Answer from the drawing. Dimensions are ordinates in mm from the lowest x, y and z of the part. Give positions to 0.01 mm unless a question says otherwise; leave off trailing zeros. Order: outer loops, then holes, each group sorted by start corner. A loop starts at its lowest first (then second) coordinate and runs counter-clockwise, first axis right, second up.
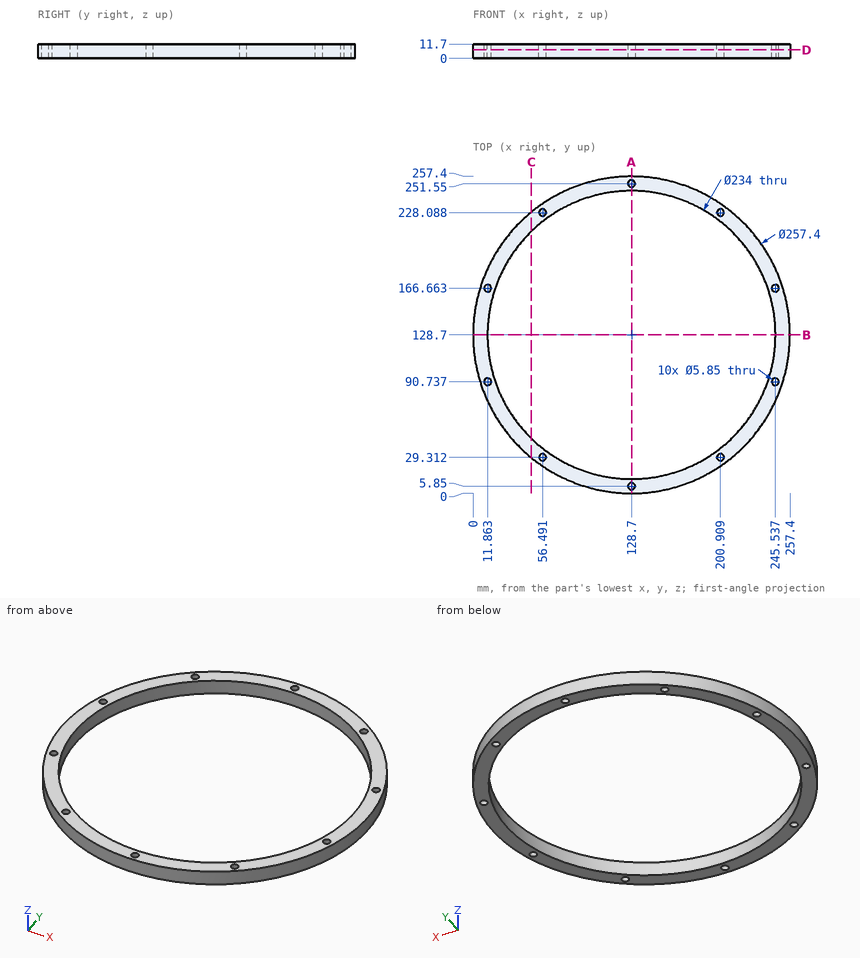
1) The part is cut by section B-B on y = 128.7. Determine the outline of the cut face in (x, z).
Final values:
outline: (0, 0) - (11.7, 0) - (11.7, 11.7) - (0, 11.7) - close; (245.7, 0) - (257.4, 0) - (257.4, 11.7) - (245.7, 11.7) - close
2) The part is cut by section A-A on x = 128.7. Determine the outline of the cut face in (y, z) (1 decimal).
Final values:
outline: (0, 0) - (2.9, 0) - (2.9, 11.7) - (0, 11.7) - close; (8.8, 0) - (11.7, 0) - (11.7, 11.7) - (8.8, 11.7) - close; (245.7, 0) - (248.6, 0) - (248.6, 11.7) - (245.7, 11.7) - close; (254.5, 0) - (257.4, 0) - (257.4, 11.7) - (254.5, 11.7) - close
3) The part is cut by section C-C on x = 47.5. Determine the outline of the cut face in (y, z) (1 decimal).
Final values:
outline: (28.8, 0) - (44.5, 0) - (44.5, 11.7) - (28.8, 11.7) - close; (212.9, 0) - (228.6, 0) - (228.6, 11.7) - (212.9, 11.7) - close
4) Given pin 1 (1 mm diameter, centred on x = 230.5, z = 7.5, fed in from -Y) (1 decimal); pin 2 (5 mm diameter, centred on y = 123, z = 3.5, fed in from +X); pin 3 (1 mm diameter, centred on y = 222, z = 6.5, fed in from -X), each flat-ended and moving along its own axis, determine where each tip first touches the part or whether it passes through.
Final values:
pin 1: stops at y = 49.3
pin 2: stops at x = 257.36
pin 3: stops at x = 39.53
5) The part is cut by section D-D on z = 7. Count the separate pieces of the cut face and the enclosed holes in it, and give its area (3 significant figures).
Final values:
separate pieces: 1
enclosed holes: 11
area: 8,760 mm2
6) Consider L1, parallel to Y at x = 128.7, z = 7 (1 decimal); L2, parallel to X at y = 88.5, z = 5.5 (1 decimal); L3, parallel to X at y = 89, z = 3.75 (1 decimal). Determine where each line is inside the solid, lowest interval first.
Final values:
L1: y = 0 to 2.9, 8.8 to 11.7, 245.7 to 248.6, 254.5 to 257.4
L2: x = 6.4 to 10, 13.7 to 18.8, 238.6 to 243.7, 247.4 to 251
L3: x = 6.3 to 9.5, 14.2 to 18.6, 238.8 to 243.2, 247.9 to 251.1
